Drawing for the job (mm, zero at the part's lowest x, y, z). A direction names the side the tool comes from. Round coordinates to 2 decimals unless told otherwise and drop trailing zeros. Order: outer loops, then holes, each group sorted by start corner. A loop starts at its lowest first (then second) coordinate and runs counter-clockwise, first axis right, second up. Notation, with made-up numbers: (69, 59.5) - (114, 59.5) arc R29 ccw to (114, 93.5) - close; hole circle Ø10 at (-23, -39). An arc over 180 degrees is marked (long way). Put each result on its own line as item: value. Start each with the question number.
Item 1: Saw through at A-A on y = 31.75. List the corners of the cut face in (x, z) (1 decimal), plus the area to 3 significant figures.
Item 2: Mould opens along Y. For the marked faces 3, 4 and 5 say: pulls with the +Y half, pulls with the -Y half, needs draft (parallel to the pull), parting line crosses it, or undercut.
Item 3: Saw through at B-B on x = 31.75. List the corners of the cut face in (y, z) (1 decimal).
Item 4: Which spindle directions (+Z, -Z, +X, -X, +Y, -Y) get a long thin tool onto all of the face, cutting with end or side? Do the marked faces 1 and 2. Say none if no direction does.
Item 5: Saw through at D-D on y = 10.5. List the corners of the cut face in (x, z), plus the area to 3 significant figures.
Item 6: Probe probe 1 along X at (y, z) = (31.75, 8.25) (1 decimal); probe 2 along X at (y, z) = (31.75, 2.5) (1 decimal); probe 3 along Y at (x, z) = (31.75, 7) (1 decimal). List the from-to ranges inside material, lowest first.
Item 7: Pin check, flat tips, straight feed: pin 1 Ø3 at (y, z) = (51.5, 2) entering from +X; pin 2 Ø2 at (y, z) = (49, 3.5) entering from -X; pin 3 Ø3 at (x, z) = (20.5, 6) entering from +Y; pin 4 Ø6 at (x, y) = (47.5, 50.5) entering from +Z. Stop position of each tip, or through.
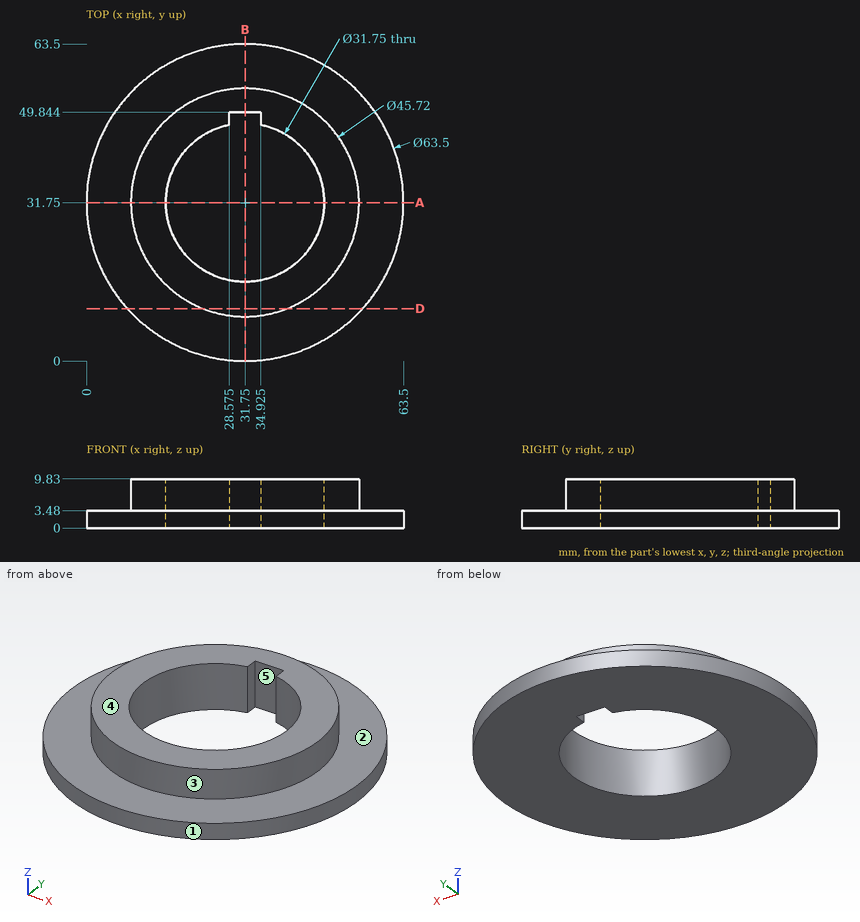
Results found:
1. outline: (0, 0) - (15.9, 0) - (15.9, 9.8) - (8.9, 9.8) - (8.9, 3.5) - (0, 3.5) - close; (47.6, 0) - (63.5, 0) - (63.5, 3.5) - (54.6, 3.5) - (54.6, 9.8) - (47.6, 9.8) - close
1. area: 199 mm²
2. face 3: parting line crosses it
2. face 4: needs draft
2. face 5: undercut
3. outline: (0, 0) - (15.9, 0) - (15.9, 9.8) - (8.9, 9.8) - (8.9, 3.5) - (0, 3.5) - close; (49.8, 0) - (63.5, 0) - (63.5, 3.5) - (54.6, 3.5) - (54.6, 9.8) - (49.8, 9.8) - close
4. face 1: +Z, -Z
4. face 2: +Z
5. outline: (8.16, 0) - (55.34, 0) - (55.34, 3.48) - (40.18, 3.48) - (40.18, 9.83) - (23.32, 9.83) - (23.32, 3.48) - (8.16, 3.48) - close
5. area: 271 mm²
6. probe 1: x = 8.9 to 15.9, 47.6 to 54.6
6. probe 2: x = 0 to 15.9, 47.6 to 63.5
6. probe 3: y = 8.9 to 15.9, 49.8 to 54.6
7. pin 1: stops at x = 57.73
7. pin 2: stops at x = 4.47
7. pin 3: stops at y = 52.43
7. pin 4: stops at z = 9.83
